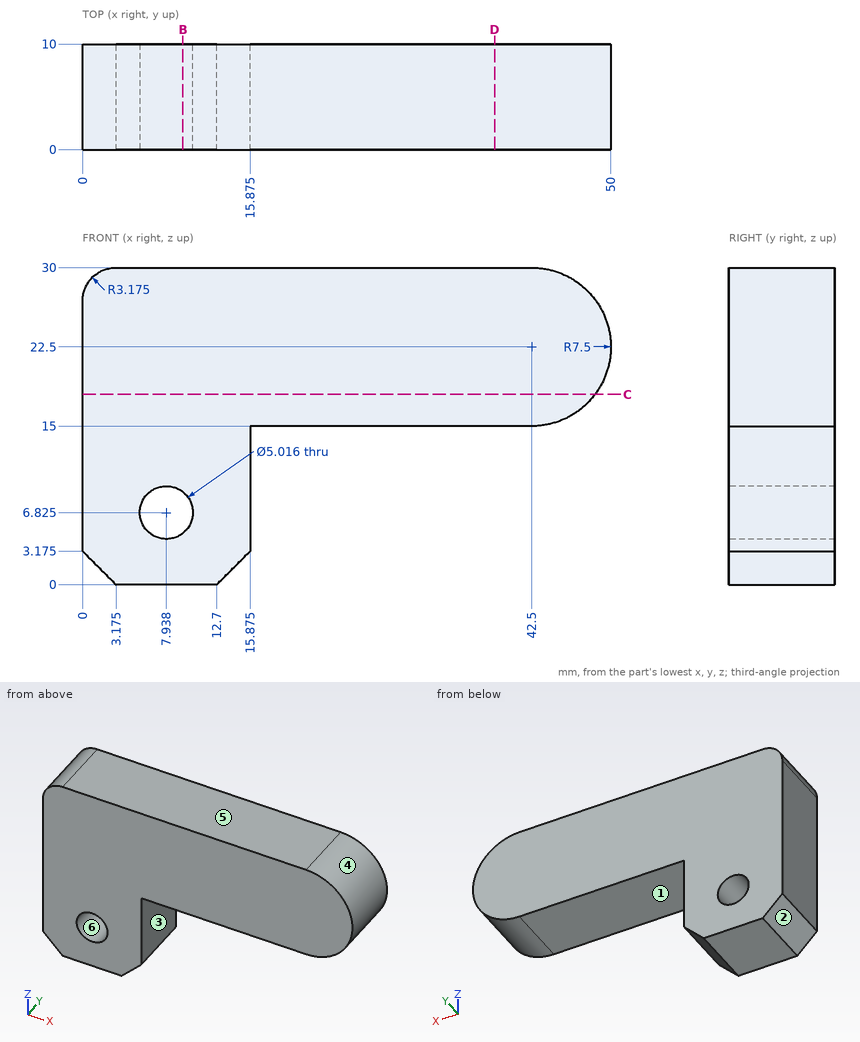
Geometry: see drawing. Coordinates: mm, zero at the bounding-box minimum. A direction names the side the tool comes from. Coordinates: 2 decimals unless noted, no trailing zeros. Loops run counter-clockwise (first coordinate to the right, second up) from the corner with the lowest first, then second, coordinate; pieces in that order, holes last.
(1) Section B-B on x = 9.5. Return the cut outline in (y, z), then the cut area to 3 significant figures.
(2) Set-up query: the marked faces 1 and 2. Return all of +Z, -Z, +X, -X, +Y, -Y with unobstructed straight access to the full face (end or side cutting, diameter ignored); none if empty.
(3) Section C-C on z = 18. Return the cut outline in (x, y).
(4) Material intervals for probe 1 along Z at (x, y) = (41, 6.75); probe 2 along X at (y, z) = (3, 8) (1 decimal); probe 3 along X at (y, z) = (1.25, 14) (1 decimal), sorted ascending.
(5) Pull-direction query (Z, two-part tool) for the marked faces 3, 4, 5 and 6; classes: released by +Z, released by -Z, zero draft, split by the parting line, or undercut.
(6) Section D-D on x = 39. Return the cut outline in (y, z), then the cut area to 3 significant figures.
(7) First-contact query: pin 1 Ø1.5 at (y, z) = (9, 8) entering from +X (1 decimal); pin 2 Ø3 at (x, y) = (30.5, 3.5) entering from -Z; pin 3 Ø8 at (x, z) = (7.94, 6.82) entering from -Y. Flat tips, straight axial feed; report the tip coordinate or a pass-through.
Data:
1. outline: (0, 0) - (10, 0) - (10, 4.86) - (0, 4.86) - close; (0, 8.79) - (10, 8.79) - (10, 30) - (0, 30) - close
1. area: 261 mm2
2. face 1: -Z, +X, +Y, -Y
2. face 2: -Z, -X, +Y, -Y
3. outline: (0, 0) - (48.5, 0) - (48.5, 10) - (0, 10) - close
4. probe 1: z = 15 to 30
4. probe 2: x = 0 to 5.7, 10.2 to 15.9
4. probe 3: x = 0 to 15.9
5. face 3: zero draft
5. face 4: split by the parting line
5. face 5: released by +Z
5. face 6: undercut
6. outline: (0, 15) - (10, 15) - (10, 30) - (0, 30) - close
6. area: 150 mm2
7. pin 1: stops at x = 15.9
7. pin 2: stops at z = 15
7. pin 3: stops at y = 0
